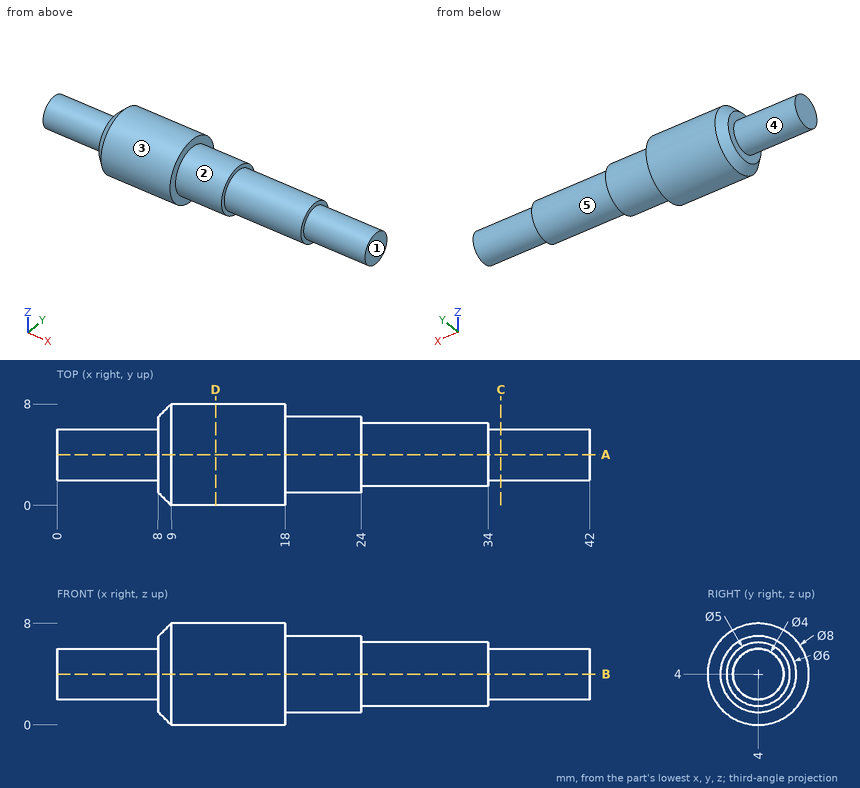
Job drawing, mm, ordinate dimensions from the low corner. One solid piece. A direction names the side the tool comes from. Give positions to 0.01 mm unless a question says otherwise; leave off trailing zeros. Write each loop counter-clockwise with the first axis right and the second up, starting at its lowest first coordinate (ties: lowest second). Pieces come first, ordered by that corner, then holes. Notation, with made-up numbers: M -9,3 L 24,3 A30 ccw 24,32 Z; hole C 47,21.25 d1. An arc over 180 degrees is marked long. One line per item, written item: value. Start each with the question number.
Q1. Two-plate mould, pull along Z, no slides. Class the marked faces 1 and 2: +Z half, -Z half, draft (parallel to the pull), parting line (faces both ways), or undercut.
Q2. Saw through at D-D, the plane x = 12.5. Write the cut outline in (y, z).
Q3. Drop flat-ended pins along their axis: pin 1 Ø3 at (x, z) = (20.5, 2) entering from -Y; pin 2 Ø4 at (x, y) = (28, 2.5) entering from -Z; pin 3 Ø2 at (x, z) = (25.5, 5.5) entering from -Y. Give the stop position or say it passes through.
Q4. Saw through at A-A, the plane y = 4. Write the cut outline in (x, z), plus the area to 3 significant figures.
Q5. Probe probe 1 along X at (y, z) = (6.5, 3); probe 2 along Z at (x, y) = (24.5, 3.5); probe 3 along Y at (x, z) = (3.5, 3). List the from-to ranges inside material, lowest first. Write a range as [from, to].
Q6. 3-axis set-ups, long thin cutter, end or side, ignore diameter. For the marked faces 3, 4 and 5: which of +Z, -Z, +X, -X, +Y, -Y reach the whole face in a straight line?
Q7. Saw through at C-C, the plane x = 35. Write the cut outline in (y, z).
Output values:
1. face 1: draft
1. face 2: parting line
2. outline: C 4,4 d8
3. pin 1: stops at y = 1.04
3. pin 2: stops at z = 1.5
3. pin 3: stops at y = 1.55
4. outline: M 0,2 L 8,2 L 8,1 L 9,0 L 18,0 L 18,1 L 24,1 L 24,1.5 L 34,1.5 L 34,2 L 42,2 L 42,6 L 34,6 L 34,6.5 L 24,6.5 L 24,7 L 18,7 L 18,8 L 9,8 L 8,7 L 8,6 L 0,6 Z
4. area: 229 mm²
5. probe 1: x = [8, 24]
5. probe 2: z = [1.55, 6.45]
5. probe 3: y = [2.27, 5.73]
6. face 3: +X, -X
6. face 4: -X
6. face 5: +X
7. outline: C 4,4 d4
